Here's how the part is built. I have some questions about the finished solid (model axes, mm). Face numbers are marked on the shaded views. A direction names the side the tool comes from. Round coordinates to 2 decimals unless told otherwise and drop trailing zeros. Loops run counter-clockwise (first coordinate to the right, second up) from the corner with the lowest first, then second, coordinate; pieces in that order, holes last. Notation, with made-up numbers: M -30.75,66.5 L -6.75,66.5 A14 cw -6.75,85.5 Z; hole C 35,42.25 d2. An arc over 180 degrees is marked long. Answer as a JSON object with one key per item and string values.
Autodesk Inventor part; units mm, degrees
ref_plane "YZ Plane" through (0, 0, 0) normal (1, 0, 0) x (0, 1, 0)
ref_plane "XZ Plane" through (0, 0, 0) normal (0, 1, 0) x (-1, 0, 0)
ref_plane "XY Plane" through (0, 0, 0) normal (0, 0, 1) x (1, 0, 0)
sketch "Sketch2" plane through (0, 0, 0) normal (1, 0, 0) x (0, 1, 0)
  line L0 (0, 6) -> (18, 6)
  line L1 (18, 6) -> (18, 4.5)
  line L2 (18, 4.5) -> (13.5, 4.5)
  line L3 (13.5, 4.5) -> (13.5, -4.5)
  line L4 (13.5, -4.5) -> (18, -4.5)
  line L5 (18, -4.5) -> (18, -6)
  line L6 (18, -6) -> (0, -6)
  line L7 (0, -6) -> (0, 6)
  point P0 (0, 0)
  point P1 (18, -5.25)
  dimension "d0" = 18
  dimension "d1" = 4.5
  dimension "d2" = 18
  dimension "d3" = 12
  dimension "d4" = 6
  dimension "d5" = 1.5
revolve "Revolution1" add sketch "Sketch2" angle 360 about axis through (0, 0, -6) along (0, 0, 1)
sketch "Sketch3" plane through (0, 0, 6) normal (0, 0, 1) x (1, 0, 0)
  arc A0 (-2, -1.5) -> (-2, 1.5) centre (0, 0) ccw
  line L0 (-2, 1.5) -> (-2, -1.5)
  point P0 (0, 0)
  dimension "d14" = 5
  dimension "d15" = 3
extrude "Extrusion1" cut sketch "Sketch3" against normal through all
properties part number "Pulley"
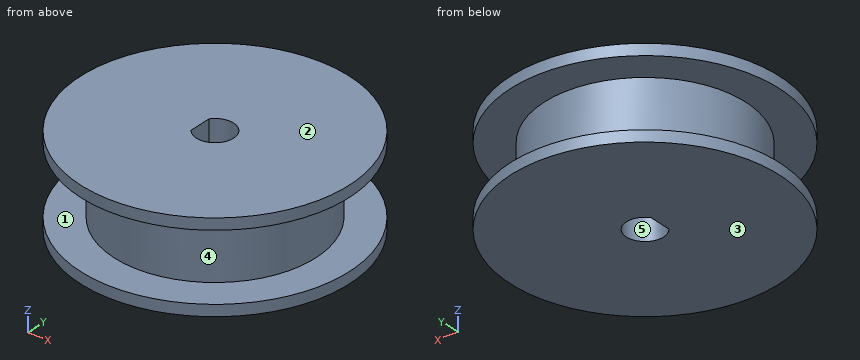
Item 1: I want a section at C-C, the plane z = -0.75. Please give me the cut outline in (x, y), then the cut area to 3 significant figures.
Resolved:
{"outline": "C 0,0 d27; hole M -2,-1.5 A2.5 ccw long -2,1.5 Z", "area": "554 mm²"}
Item 2: I want a section at B-B, the plane y = 0. Please give me the cut outline in (x, z), then the cut area to 3 significant figures.
Resolved:
{"outline": "M -18,-6 L -2,-6 L -2,6 L -18,6 L -18,4.5 L -13.5,4.5 L -13.5,-4.5 L -18,-4.5 Z; M 2.5,-6 L 18,-6 L 18,-4.5 L 13.5,-4.5 L 13.5,4.5 L 18,4.5 L 18,6 L 2.5,6 Z", "area": "297 mm²"}
Item 3: If we mould it in two halves opening along X, with no side actions, what happens to the marked faces 3, 4 and 5? For each: pulls with the +X half, pulls with the -X half, needs draft (parallel to the pull), parting line crosses it, or undercut.
Resolved:
{"face 3": "needs draft", "face 4": "parting line crosses it", "face 5": "undercut"}
Item 4: I'm going to push flat-ended pins straight in: pin 1 Ø8 at (x, y) = (0, 0) entering from +Z; pin 2 Ø6 at (y, z) = (9, 0.5) entering from +X; pin 3 Ø1 at (x, z) = (5.5, 0.5) entering from +Y; pin 4 Ø1 at (y, z) = (-10, -0.5) entering from -X. Where does each tip first touch, or does it pass through?
Resolved:
{"pin 1": "z = 6", "pin 2": "x = 12.09", "pin 3": "y = 12.54", "pin 4": "x = -9.59"}
Item 5: I want a section at D-D, the plane y = -11.5. Please give me the cut outline in (x, z), then the cut area to 3 significant figures.
Resolved:
{"outline": "M -13.85,-6 L 13.85,-6 L 13.85,-4.5 L 7.07,-4.5 L 7.07,4.5 L 13.85,4.5 L 13.85,6 L -13.85,6 L -13.85,4.5 L -7.07,4.5 L -7.07,-4.5 L -13.85,-4.5 Z", "area": "210 mm²"}
Item 6: On a 3-axis mill with a long thin cutter (end or side, diameter ignored), from which of +Z, -Z, +X, -X, +Y, -Y can I reach the whole of each face in a straight line? I mean the marked faces 1 and 2. Say none if no direction works.
Resolved:
{"face 1": "none", "face 2": "+Z, +X, -X, +Y, -Y"}
Item 7: Please list where these lines run through material, in increasing order: probe 1 along Z at (x, y) = (15.5, 4.5); probe 2 along X at (y, z) = (0, -2); probe 3 along Y at (x, z) = (0, 1). Write a range as from..to.
Resolved:
{"probe 1": "-6..-4.5, 4.5..6", "probe 2": "-13.5..-2, 2.5..13.5", "probe 3": "-13.5..-2.5, 2.5..13.5"}
Item 8: I want a section at A-A, the plane x = 0. Please give me the cut outline in (y, z).
Resolved:
{"outline": "M -18,-6 L -2.5,-6 L -2.5,6 L -18,6 L -18,4.5 L -13.5,4.5 L -13.5,-4.5 L -18,-4.5 Z; M 2.5,-6 L 18,-6 L 18,-4.5 L 13.5,-4.5 L 13.5,4.5 L 18,4.5 L 18,6 L 2.5,6 Z"}
